Study the drawing (mm; zero at the part's minimum x, y, z) and answer. Round coordinates to 2 decimals unless told otherwise and drop trailing zeros. Order: outer loops, then holes, each group sorted by start corner. A loop starts at its lowest first (then second) coordinate and runs counter-clockwise, first axis right, second up. Notation, with made-up numbers: (-9.5, 31) - (43.5, 31) arc R20 cw to (43.5, 46) - close; hole circle Ø4 at (-31, 17.5). An arc over 180 degrees is marked (long way). Put each result on its own line as item: value. Start each with the question number.
Q1. Find the intervals of material crossed by line 1 along Z through (x, y) = (5.5, 40.5); line 2 along Z through (x, y) = (7, 22); line 3 along Y through (x, z) = (4, 42), in increasing order. Write a range as from..to.
Q2. Section A-A on x = 9.5 is taken. Give the vertices of the cut face in (y, z).
Q3. Section B-B on x = 6 is taken. Give the vertices of the cut face in (y, z).
Q4. Each of these flat-tipped pins is pushed along its axis until it touches: pin 1 Ø5 at (x, z) = (20.5, 34.5) entering from -Y; pin 2 Ø6 at (x, z) = (6, 38) entering from -Y; pin 3 Ø3 at (y, z) = (33.5, 43) entering from +X; pin 4 Ø2 at (y, z) = (31.5, 32.5) entering from +X. Where does it stop, or does it pass through?
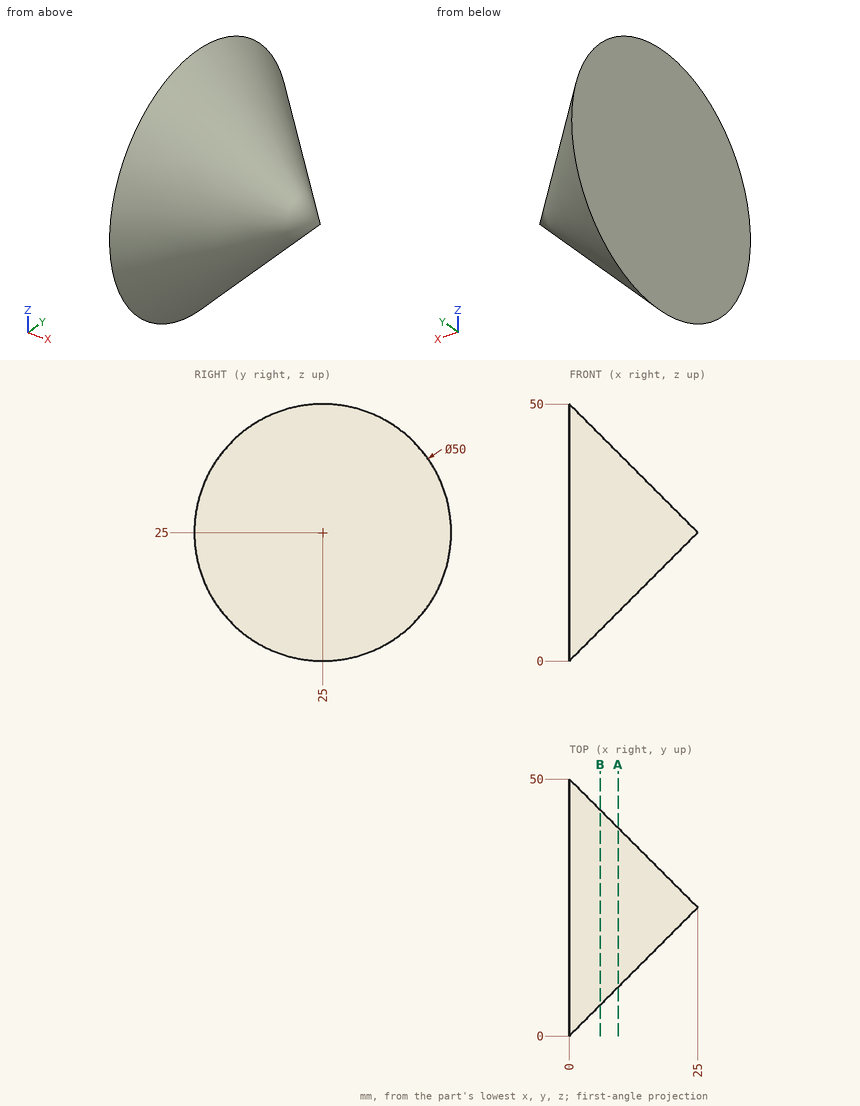
Findings:
1. line 1: 13.17..36.83
1. line 2: 7.25..42.75
1. line 3: 12.67..37.33
2. outline: circle Ø31 at (25, 25)
3. outline: circle Ø38 at (25, 25)
4. pin 1: through
4. pin 2: y = 6.72
4. pin 3: x = 6.59
4. pin 4: x = 16.08
